CAD build for the part. Positions are in the model's coordinates, mm. A direction names the side the tool comes from. Give positions to 0.01 mm unless a question says otherwise; leave off trailing zeros. Write each loop counter-clockwise with the first axis right and the second up, starting at its lowest first coordinate (ties: lowest second). Pieces come first, ordered by that corner, then holes. Notation, with made-up numbers: (-17, -13.5) - (-2, -13.5) arc R20 cw to (-2, 24.5) - close; hole circle Ø6 at (53, -34.5). An arc over 180 degrees is marked (long way). Answer as a JSON object with one key per item and string values.
from build123d import *

# Parameters (mm, degrees)
EXTRUDE_THIN1_DEPTH = 412.75
FILLET1_R           = 1.016


with BuildPart() as part:
    # Sketch1 → Extrude-Thin1 (new body)
    with BuildSketch(Plane.XY):
        Polygon((3.175, 37.703125), (3.175, 40.878125), (-15.08125, 41.275), (-14.2875, 31.75), (-10.31875, 31.75), (-8.73125, 12.7), (-4.7625, 12.7), (-3.96875, 0), (0, 0), (-0.396875, 12.7), (-1.412379269, 12.668265492), (-1.048245973, 1.016), (-3.014267559, 1.016), (-3.808017559, 13.716), (-7.796394992, 13.716), (-9.383894992, 32.766), (-13.352644992, 32.766), (-13.975037647, 40.234711858), (2.159, 39.883971909), (2.159, 37.703125), align=None)
    extrude(amount=-EXTRUDE_THIN1_DEPTH)

    # Fillet1
    fillet1_edges = [part.edges().sort_by_distance(p)[0] for p in [
        (-9.383894992, 32.766, -206.375),
        (-3.808017559, 13.716, -206.375),
        (0, 0, -206.375),
        (-3.96875, 0, -206.375),
        (-8.73125, 12.7, -206.375),
        (-14.2875, 31.75, -206.375),
        (-15.08125, 41.275, -206.375),
        (3.175, 40.878125, -206.375),
    ]]
    fillet(fillet1_edges, radius=FILLET1_R)


solid = part.part
(1) Pull direction Y, two halves, no side cores. Call faces 1 (the face through (-3.376, 6.807, -203.486)), 2 (the face through (-9, 24, 0)), 3 (the face through (-8.54, 22.65, -203.49)), 4 (the face through (-9.574, 22.818, -203.486)): pulls with the +Y half, pulls with the -Y half, needs draft (parallel to the pull), parting line crosses it, or undercut.
Answer key:
{"face 1": "undercut", "face 2": "needs draft", "face 3": "undercut", "face 4": "pulls with the -Y half"}
(2) Flat gauge pins, fed straight in: P1, Ø0.9, axis at x = -12, z = -249, coming from the +Y side; P2, Ø1.7, axis at y = 38.5, z = -104.5, coming from the -X side; P3, Ø1, axis at y = 16, z = -127, coming from the -X side. Where does each tip first touch, or does it go through?
Answer key:
{"P1": "stops at y = 41.22", "P2": "stops at x = -14.92", "P3": "stops at x = -9.05"}
(3) Probe L1, parallel to Y at x = -13, z = -187; L2, parallel to Y at x = -12, z = -330.5; L3, parallel to X at y = 32, z = -71. List the from-to ranges inside material, lowest first. Write a range as [from, to].
Answer key:
{"L1": "y = [31.75, 32.77], [40.21, 41.23]", "L2": "y = [31.75, 32.77], [40.19, 41.21]", "L3": "x = [-14.02, -9.33]"}
(4) Saw through at B-B, the plane y = 8. Give the cut face in (x, z), and give its area (3 significant figures).
Answer key:
{"outline": "(-4.47, -412.75) - (-3.45, -412.75) - (-3.45, 0) - (-4.47, 0) - close; (-1.27, -412.75) - (-0.25, -412.75) - (-0.25, 0) - (-1.27, 0) - close", "area": "840 mm²"}
(5) Saw through at C-C, the plane y = 28. Give the cut face in (x, z).
Answer key:
{"outline": "(-10.01, -412.75) - (-8.99, -412.75) - (-8.99, 0) - (-10.01, 0) - close"}
(6) 3-axis set-ups, long thin cutter, end or side, ignore diameter. For faces 5 (the face through (-9, 24, -412.75)), 6 (the face through (-13.66, 36.45, -203.49)): which of +Z, -Z, +X, -X, +Y, -Y reach the whole face in a straight line?
Answer key:
{"face 5": "-Z, +X, -X, +Y, -Y", "face 6": "+Z, -Z"}
